Input: part model. Units: mm. Frame: model coordinates. Face numbers are marked on the shaded views. A direction names the side the tool comes from. Coordinates: 2 decimals unless noted, no trailing zeros. Loops run counter-clockwise (first coordinate to the right, second up) from the corner with the lowest first, then second, coordinate; pieces in that order, holes last. Notation, with made-up numbers: (62, -16) - (90, -16) arc R31 ccw to (90, 17) - close; hole circle Ø4 at (73, -14.5). An arc over 180 degrees is marked (long way). Use one line per item in the form item = value.
Autodesk Inventor part; units mm, degrees
ref_plane "YZ Plane" through (0, 0, 0) normal (1, 0, 0) x (0, 1, 0)
ref_plane "XZ Plane" through (0, 0, 0) normal (0, 1, 0) x (-1, 0, 0)
ref_plane "XY Plane" through (0, 0, 0) normal (0, 0, 1) x (1, 0, 0)
sketch "Sketch1" plane through (0, 0, 0) normal (0, 1, 0) x (-1, 0, 0)
  line L0 (33.9701, -0.003) -> (69.9315, -0.003)
  line L1 (69.9315, -0.003) -> (69.9315, -52.003)
  line L2 (69.9315, -52.003) -> (-0.0685, -52.003)
  line L3 (-0.0685, -49.003) -> (69.9315, -49.003)
  line L4 (34.9315, -3.003) -> (69.9315, -3.003)
  line L5 (-0.0685, -28.003) -> (34.9315, -3.003)
  line L6 (29.7701, -3.003) -> (-0.0685, -24.3163)
  line L7 (-0.0685, -52.003) -> (-0.0685, -24.3163)
  line L8 (29.7701, -3.003) -> (33.9701, -0.003)
  point P0 (0, 0)
  dimension "d0" = 70
  dimension "d1" = 52
  dimension "d2" = 3
  dimension "d3" = 3
  dimension "d4" = 3
  dimension "d5" = 21
extrude "Extrusion1" add sketch "Sketch1" against normal blind 19 contours L0 L1 L4 L5 L7 L6 L8 | L1 L2 L7 L3
extrude "Extrusion2" add sketch "Sketch1" against normal blind 3 contours L1 L3 L7 L5 L4
properties part number "Cooling Fan Shroud"
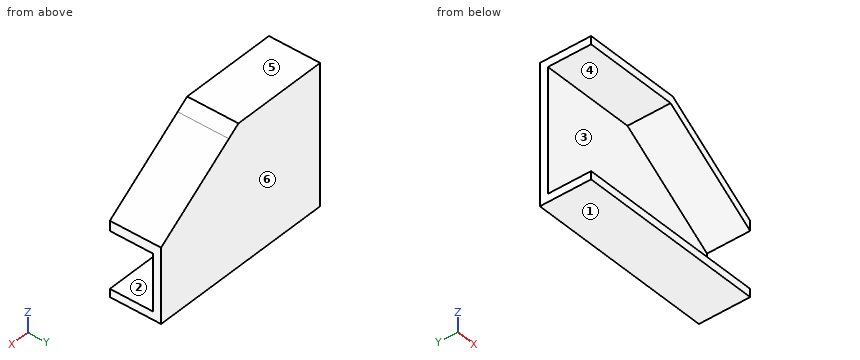
Q1. Cut plane C-C, the plane z = -42. Return loops of the section in (x, y), then the cut area to 3 significant figures.
Check values:
outline = (-69.93, -3) - (0.07, -3) - (0.07, 0) - (-69.93, 0) - close
area = 210 mm²
Q2. Ray query, line 1 along Z through (x, y) = (-40.5, -9.75); line 2 along Y through (x, z) = (-64.5, -28); line 3 along Z through (x, y) = (-34.5, -12.5). Return the intervals inside material, ascending. Write a range as [from, to].
Check values:
line_1 = [-52, -49], [-3, 0]
line_2 = [-3, 0]
line_3 = [-52, -49], [-3.31, 0]
Q3. First-contact query: P1, Ø8, axis at x = -29.5, y = -10.5, coming from the +Z side; P2, Ø1, axis at x = -13.5, z = -30, coming from the +Y side; P3, Ø8, axis at y = -11.5, z = -31.5, coming from the -X side; P4, Ø1, axis at x = -14.5, y = -10, coming from the +Z side. Flat tips, straight axial feed; report the tip coordinate or a pass-through.
Check values:
P1 = -0.34
P2 = 0
P3 = -0.64
P4 = -13.55
Q4. Cut plane D-D, the plane x = -23. Return loops of the section in (y, z).
Check values:
outline = (-19, -52) - (0, -52) - (0, -7.84) - (-19, -7.84) - (-19, -11.53) - (-3, -11.53) - (-3, -49) - (-19, -49) - close
Q5. Pull-direction query (Z, two-part tool) for the marked faces 4, 5 and 6; classes: pulls with the +Z half, pulls with the -Z half, needs draft (parallel to the pull), parting line crosses it, or undercut.
Check values:
face_4 = undercut
face_5 = pulls with the +Z half
face_6 = needs draft
Q6. Cut plane A-A, the plane y = -12. Return loops of the section in (x, z).
Check values:
outline = (-69.93, -52) - (0.07, -52) - (0.07, -49) - (-69.93, -49) - close; (-69.93, -3) - (-34.93, -3) - (0.07, -28) - (0.07, -24.32) - (-29.77, -3) - (-33.97, 0) - (-69.93, 0) - close
Q7. Cut plane B-B, the plane x = -46. Return loops of the section in (y, z), then the cut area to 3 significant figures.
Check values:
outline = (-19, -52) - (0, -52) - (0, 0) - (-19, 0) - (-19, -3) - (-3, -3) - (-3, -49) - (-19, -49) - close
area = 252 mm²
Q8. Set-up query: the marked faces 1, 2 and 3. Return all of +Z, -Z, +X, -X, +Y, -Y with unobstructed straight access to the full face (end or side cutting, diameter ignored); none if empty.
Check values:
face_1 = -Z, +X, -X, +Y, -Y
face_2 = +X, -X, -Y
face_3 = -X, -Y
